The model under review builds one solid part; all positions refer to its coordinate system, in mm. A direction names the side the tool comes from. Coordinates: 2 decimals unless noted, no trailing zeros. Order: outer loops, then holes, each group sorted by start corner. A loop starts at its lowest first (then second) coordinate and runs counter-clockwise, first axis right, second up. Notation, with made-up numbers: (-32, 72) -> (-21, 72) arc R13 cw to (-21, 85) -> close; hole circle Ø10 at (27, 34). An arc over 180 degrees is marked (long way). Put each result on its own line as item: value.
Autodesk Inventor part; units mm, degrees
ref_plane "YZ Plane" through (0, 0, 0) normal (1, 0, 0) x (0, 1, 0)
ref_plane "XZ Plane" through (0, 0, 0) normal (0, 1, 0) x (-1, 0, 0)
ref_plane "XY Plane" through (0, 0, 0) normal (0, 0, 1) x (1, 0, 0)
sketch "Boceto1" plane through (0, 0, 0) normal (0, 1, 0) x (-1, 0, 0)
  line L0 (41.275, 139.7) -> (0, 139.7)
  line L1 (0, 139.7) -> (0, 0)
  line L2 (0, 0) -> (41.275, 0)
  line L3 (41.275, 0) -> (41.275, 139.7)
  dimension "d0" = 139.7
  dimension "d1" = 41.275
extrude "Extrusión1" add sketch "Boceto1" along normal blind 5
sketch "Boceto2" plane through (0, 5, 0) normal (0, 1, 0) x (1, 0, 0)
  circle A0 centre (-22.225, -122.2375) radius 5
  line L0 (-41.275, -139.7) -> (0, -139.7)
  circle A1 centre (-22.225, -126.9609) radius 5
  circle A2 centre (-22.225, -117.5141) radius 5
  line L1 (-22.225, -126.9609) -> (-22.225, -122.2375)
  line L2 (-22.225, -122.2375) -> (-22.225, -117.5141)
  line L3 (-41.275, -139.7) -> (-41.275, 0)
  line L4 (-17.225, -126.9609) -> (-17.225, -117.5141)
  line L5 (-27.225, -126.9609) -> (-27.225, -117.5141)
  circle A3 centre (-22.225, -17.4625) radius 5
  circle A4 centre (-22.225, -22.1859) radius 5
  circle A5 centre (-22.225, -12.7391) radius 5
  line L6 (-22.225, -22.1859) -> (-22.225, -17.4625)
  line L7 (-22.225, -17.4625) -> (-22.225, -12.7391)
  line L8 (0, 0) -> (-41.275, 0)
  line L9 (-27.225, -22.1859) -> (-27.225, -12.7391)
  line L10 (-17.225, -22.1859) -> (-17.225, -12.7391)
  dimension "d4" = 10
  dimension "d5" = 17.4625
  dimension "d6" = 10
  dimension "d7" = 10
  dimension "d8" = 19.4469
  dimension "d9" = 19.05
  dimension "d10" = 10
  dimension "d11" = 10
  dimension "d12" = 10
  dimension "d13" = 19.4469
  dimension "d14" = 19.05
  dimension "d15" = 17.4625
extrude "Extrusión2" cut sketch "Boceto2" against normal up to next
fillet "Empalme1" radius 4.7625 4 edges at (0, 2.5, 139.7) (-41.275, 2.5, 139.7) (0, 2.5, 0) (-41.275, 2.5, 0)
properties part number "CAR LATERAL BEARING HOLDER"
Item 1: For line 1 (Z direction, x = -23, y = 4.65); line 2 (X direction, y = 3.35, z = 15.5) (3 decimals); line 3 (Z direction, x = -3, y = 3.2), list the stretches that pass through material, from the lowest coordinate up. Write a range as from..to.
Answers below:
line 1: 0..7.8, 27.13..112.57, 131.9..139.7
line 2: -41.275..-27.225, -17.225..0
line 3: 0.34..139.36
Item 2: Consider section C-C on x = -21.5. Write out the cut boundary in (y, z), and give its area (3 significant figures).
Answers below:
outline: (0, 0) -> (5, 0) -> (5, 7.79) -> (0, 7.79) -> close; (0, 27.13) -> (5, 27.13) -> (5, 112.57) -> (0, 112.57) -> close; (0, 131.91) -> (5, 131.91) -> (5, 139.7) -> (0, 139.7) -> close
area: 505 mm^2
Item 3: Mouldability with a two-part tool opening along X and no side actions: class faces 1 (the cylindrical face through (-22.33, 2.54, 131.96)), 2 (the flat face through (-21, 2, 139.7)), 3 (the flat face through (0, 2, 71)) as +X half, -X half, draft (parallel to the pull), parting line (faces both ways), or undercut.
Answers below:
face 1: undercut
face 2: draft
face 3: +X half
Item 4: Consider section D-D on z = 115. Write out the cut boundary in (x, y) (3 decimals).
Answers below:
outline: (-41.275, 0) -> (-26.547, 0) -> (-26.547, 5) -> (-41.275, 5) -> close; (-17.903, 0) -> (0, 0) -> (0, 5) -> (-17.903, 5) -> close
Item 5: Consider section B-B on z = 16.5. Write out the cut boundary in (x, y) (3 decimals).
Answers below:
outline: (-41.275, 0) -> (-27.225, 0) -> (-27.225, 5) -> (-41.275, 5) -> close; (-17.225, 0) -> (0, 0) -> (0, 5) -> (-17.225, 5) -> close
Item 6: Consider section A-A on y = 3.65. Write out the cut boundary in (x, z) (1 decimal).
Answers below:
outline: (-41.3, 4.8) arc R4.8 ccw to (-36.5, 0) -> (-4.8, 0) arc R4.8 ccw to (0, 4.8) -> (0, 134.9) arc R4.8 ccw to (-4.8, 139.7) -> (-36.5, 139.7) arc R4.8 ccw to (-41.3, 134.9) -> close; hole (-27.2, 12.7) arc R5 ccw to (-17.2, 12.7) -> (-17.2, 22.2) arc R5 ccw to (-27.2, 22.2) -> close; hole (-27.2, 117.5) arc R5 ccw to (-17.2, 117.5) -> (-17.2, 127) arc R5 ccw to (-27.2, 127) -> close
Item 7: For faces 4 (the flat face through (-20, 0, 71)), 5 (the flat face through (-17.225, 3, 18)), list the 3-axis set-ups (+Z, -Z, +X, -X, +Y, -Y) from which the entire face can be reached by the end or side of a thin tool; tool diameter is ignored.
Answers below:
face 4: +Z, -Z, +X, -X, -Y
face 5: +Y, -Y
